Design review of the part built by this model. Coordinates are the model's own, in mm. Round coordinates to 2 decimals unless told otherwise and drop trailing zeros. Loops run counter-clockwise (first coordinate to the right, second up) from the corner with the lowest first, then second, coordinate; pieces in that order, holes last. Notation, with made-up numbers: M -33,27.5 L -29,27.5 A7 cw -29,39.5 Z; hole C 52.25,58.5 d9. An arc over 180 degrees is marked long. Answer as CSV lines item,"result". Start each with the question number.
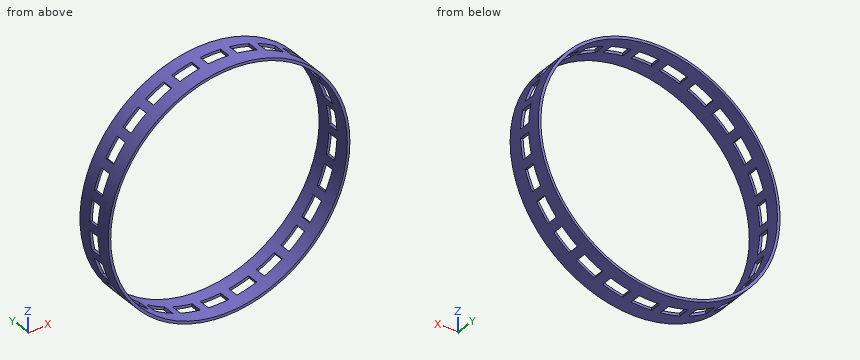
from build123d import *

# Parameters (mm, degrees)
SKETCH1_R           = 118.5
SKETCH1_R_2         = 116
BOSS_EXTRUDE1_DEPTH = 38
SKETCH2_W           = 20
SKETCH2_H           = 11
CUT_EXTRUDE1_DEPTH  = 119.5
CIRPATTERN1_COUNT   = 13


with BuildPart() as part:
    # Sketch1 → Boss-Extrude1 (new body)
    with BuildSketch(Plane(origin=(0, 0, 0), x_dir=(1, 0, 0), z_dir=(0, 1, 0))):
        Circle(SKETCH1_R)
        Circle(SKETCH1_R_2, mode=Mode.SUBTRACT)
    extrude(amount=BOSS_EXTRUDE1_DEPTH)

    # Sketch2 → Cut-Extrude1 (cut, symmetric)
    with BuildSketch(Plane.XY):
        with Locations((0, 19.5)):
            Rectangle(SKETCH2_W, SKETCH2_H)
    cut_extrude1 = extrude(amount=CUT_EXTRUDE1_DEPTH, both=True, mode=Mode.SUBTRACT)

    # CirPattern1: Cut-Extrude1 ×13 about axis
    cirpattern1_axis = Axis((0, 0, 0), (0, 1, 0))
    for i in range(1, CIRPATTERN1_COUNT):
        add(cut_extrude1.rotate(cirpattern1_axis, i * 360 / CIRPATTERN1_COUNT), mode=Mode.SUBTRACT)


solid = part.part
Item 1: Consider section B-B, the plane x = 0. Write out the cut boundary in (y, z).
Item 2: Insertion check: pin 1 Ø12 at (x, y) = (-55, 12) entering from +Z; pin 2 Ø2 at (y, z) = (20.5, 116.5) entering from +X; pin 3 Ø5 at (x, y) = (92.5, 16) entering from +Z. Each pin has a flat end and moves straight along its axis. Give the tip position at first contact, or say it passes through.
Item 3: Consider section C-C, the plane z = -44. Write out the cut boundary in (x, y).
Item 4: Consider section D-D, the plane y = 31.5. Write out the cut boundary in (x, z), then the cut area to 3 significant figures.
Item 5: To check wall thickness, follow line 1 (X direction, y = 7, z = 24); line 2 (X direction, y = 27, z = 0). State the ranges of each line that lie inside material, in increasing order.
Item 6: Consider section A-A, the plane z = 0. Write out the cut boundary in (x, y).
Found:
1,outline,"M 0,-118.5 L 14,-118.5 L 14,-116 L 0,-116 Z; M 0,116 L 14,116 L 14,118.5 L 0,118.5 Z; M 25,-118.5 L 38,-118.5 L 38,-116 L 25,-116 Z; M 25,116 L 38,116 L 38,118.5 L 25,118.5 Z"
2,pin 1,"stops at z = 107.89"
2,pin 2,"stops at x = 18.55"
2,pin 3,"stops at z = 77.09"
3,outline,"M -110.03,0 L -107.33,0 L -107.33,14 L -110.03,14 Z; M -110.03,25 L -107.33,25 L -107.33,38 L -110.03,38 Z; M 107.33,0 L 110.03,0 L 110.03,14 L 107.33,14 Z; M 107.33,25 L 110.03,25 L 110.03,38 L 107.33,38 Z"
4,outline,"C 0,0 d237; hole C 0,0 d232"
4,area,"1,840 mm^2"
5,line 1,"x = -116.04 to -113.49, 113.49 to 116.04"
5,line 2,"x = -118.5 to -116, 116 to 118.5"
6,outline,"M -118.5,0 L -116,0 L -116,38 L -118.5,38 Z; M 116,0 L 118.5,0 L 118.5,38 L 116,38 Z"
